```python
from build123d import *

# Parameters (mm, degrees)
SKETCH1_W                 = 50
SKETCH1_H                 = 55
BOSS_EXTRUDE1_DEPTH       = 2
SKETCH2_W                 = 50
SKETCH2_H                 = 2
BOSS_EXTRUDE2_DEPTH       = 45
CUT_EXTRUDE1_DEPTH        = 76.332595867
CUT_EXTRUDE1_DEPTH_BACK   = 76.332595867
SKETCH3_R                 = 1.7
LO_TAM_D22_DEPTH          = 76.332595867
LO_TAM_D22_DEPTH_BACK     = 76.332595867
SKETCH4_R                 = 11
HAI_LO_CHAN_M3_DEPTH      = 76.332595867
HAI_LO_CHAN_M3_DEPTH_BACK = 76.332595867
SKETCH5_R                 = 1.7


with BuildPart() as part:
    # Sketch1 → Boss-Extrude1 (new body)
    with BuildSketch(Plane.XY):
        with Locations((0, 27.5)):
            Rectangle(SKETCH1_W, SKETCH1_H)
    extrude(amount=-BOSS_EXTRUDE1_DEPTH)

    # Sketch2 → Boss-Extrude2 (add)
    with BuildSketch(Plane.XY):
        with Locations((0, 1)):
            Rectangle(SKETCH2_W, SKETCH2_H)
    extrude(amount=-BOSS_EXTRUDE2_DEPTH)

    # Sketch3 → Cut-Extrude1 (cut, two sides: drawn at the far end of the back side and taken through both)
    with BuildSketch(Plane.XY.offset(-CUT_EXTRUDE1_DEPTH_BACK)):
        with Locations(Location((-15.5, 19.5, 0), (0, 0, 180))):
            Circle(SKETCH3_R)
        with Locations(Location((-15.5, 50.5, 0), (0, 0, 180))):
            Circle(SKETCH3_R)
        with Locations(Location((15.5, 19.5, 0), (0, 0, 180))):
            Circle(SKETCH3_R)
        with Locations(Location((15.5, 50.5, 0), (0, 0, 180))):
            Circle(SKETCH3_R)
    extrude(amount=CUT_EXTRUDE1_DEPTH + CUT_EXTRUDE1_DEPTH_BACK, mode=Mode.SUBTRACT)

    # Sketch4 → Lo_tam_D22 (cut, two sides: drawn at the far end of the back side and taken through both)
    with BuildSketch(Plane.XY.offset(-LO_TAM_D22_DEPTH_BACK)):
        with Locations(Location((0, 35, 0), (0, 0, 180))):
            Circle(SKETCH4_R)
    extrude(amount=LO_TAM_D22_DEPTH + LO_TAM_D22_DEPTH_BACK, mode=Mode.SUBTRACT)

    # Sketch5 → Hai_lo_chan_M3 (cut, two sides: drawn at the far end of the back side and taken through both)
    with BuildSketch(Plane(origin=(0, 0, 0), x_dir=(1, 0, 0), z_dir=(0, 1, 0)).offset(-HAI_LO_CHAN_M3_DEPTH_BACK)):
        with Locations(Location((-12.5, 23, 0), (0, 0, 270))):
            Circle(SKETCH5_R)
        with Locations(Location((12.5, 23, 0), (0, 0, 270))):
            Circle(SKETCH5_R)
    extrude(amount=HAI_LO_CHAN_M3_DEPTH + HAI_LO_CHAN_M3_DEPTH_BACK, mode=Mode.SUBTRACT)


solid = part.part
```
Input: part model. Units: mm. Frame: model coordinates. Coordinates: 2 decimals unless noted, no trailing zeros. Write each loop counter-clockwise with the first axis right and the second up, starting at its lowest first coordinate (ties: lowest second). Pieces come first, ordered by that corner, then holes. Notation, with made-up numbers: M 8,28 L 23,28 A15 cw 23,42 Z; hole C 38.25,-28 d3. An arc over 180 degrees is marked long. Use one line per item in the form item = value.
Q1. Section C-C (y = 50.5). Return loops of the section in (x, z).
Answer below:
outline = M -25,-2 L -17.2,-2 L -17.2,0 L -25,0 Z; M -13.8,-2 L 13.8,-2 L 13.8,0 L -13.8,0 Z; M 17.2,-2 L 25,-2 L 25,0 L 17.2,0 Z
Q2. Section A-A (z = -23). Return loops of the section in (x, y).
Answer below:
outline = M -25,0 L -14.2,0 L -14.2,2 L -25,2 Z; M -10.8,0 L 10.8,0 L 10.8,2 L -10.8,2 Z; M 14.2,0 L 25,0 L 25,2 L 14.2,2 Z
Q3. Draft query along Y for faces 1 (the face through (0, 23, -2)), 2 (the face through (2.38, 45.74, -1.01)), 3 (the face through (0, 2, -23)). Return one class per face: released by +Y, released by -Y, zero draft, split by the parting line, or undercut.
Answer below:
face_1 = zero draft
face_2 = undercut
face_3 = released by +Y
Q4. Section D-D (x = 15.5). Return loops of the section in (y, z).
Answer below:
outline = M 0,-45 L 2,-45 L 2,-2 L 17.8,-2 L 17.8,0 L 0,0 Z; M 21.2,-2 L 48.8,-2 L 48.8,0 L 21.2,0 Z; M 52.2,-2 L 55,-2 L 55,0 L 52.2,0 Z
Q5. First-contact query: pin 1 (4.5 mm diameter, centred on x = 15.5, y = 50.5, fed in from -Z); pin 2 (3 mm diameter, centred on x = 11, z = -29.5, fed in from +Y). Flat tips, straight axial feed; report the tip coordinate or a pass-through.
Answer below:
pin_1 = -2
pin_2 = 2
Q6. Section B-B (x = 0). Return loops of the section in (y, z), plus the area to 3 significant figures.
Answer below:
outline = M 0,-45 L 2,-45 L 2,-2 L 24,-2 L 24,0 L 0,0 Z; M 46,-2 L 55,-2 L 55,0 L 46,0 Z
area = 152 mm²
Q7. Material intervals for probe 1 along X at (y, z) = (1.05, -23); probe 2 along Y at (x, z) = (15.5, -0.5); probe 3 along Y at (x, z) = (-8.5, -10.5), sorted ascending. Write a range as from..to.
Answer below:
probe_1 = -25..-14.2, -10.8..10.8, 14.2..25
probe_2 = 0..17.8, 21.2..48.8, 52.2..55
probe_3 = 0..2
